For this review, take the finished solid that the model builds, in its own axes (mm). Face numbers are marked on the shaded views. A direction names the side the tool comes from. Coordinates: 2 decimals unless noted, no trailing zeros. Write each loop counter-clockwise with the first axis right and the second up, starting at its lowest first coordinate (ties: lowest second). Pieces come first, ordered by that corner, then holes.
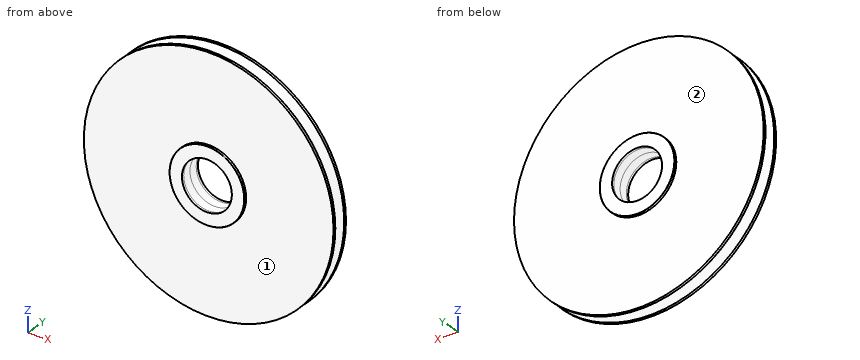
```python
from build123d import *
from build123d import SkipClean  # not in build123d's __all__

# Parameters (mm, degrees)
F0_R     = 50
F1_DEPTH = 3.5
F2_SIZE  = 2.5
F3_R     = 10.0003114876
F4_DEPTH = 3.5
F6_R     = 15
F6_R_2   = 10.0003114876
F7_DEPTH = 1
F8_R     = 15.0083101608
F8_R_2   = 10.0003114876
F9_DEPTH = 1
F10_R    = 0.1


with BuildPart() as f1:
    # F0 (on Front) → F1 (new body)
    with BuildSketch(Plane.XZ):
        Circle(F0_R)
    extrude(amount=F1_DEPTH)

    # F2
    f2_edges = [f1.edges().sort_by_distance(p)[0] for p in [
        (-50, -3.5, 0),
    ]]
    chamfer(f2_edges, length=F2_SIZE)

    # F3 (on face) → F4 (cut)
    with BuildSketch(Plane(origin=(0, 0, 0), x_dir=(-1, 0, 0), z_dir=(0, 1, 0))):
        Circle(F3_R)
    extrude(amount=-F4_DEPTH, mode=Mode.SUBTRACT)

    # F5: F1 across face


with BuildPart() as f1_1:
    add(f1.part, clean=False)
    add(f1.part.mirror(Plane.XZ.offset(3.5)), clean=False)

    # F6 (on face) → F7 (join)
    with BuildSketch(Plane.XZ.offset(7)):
        Circle(F6_R)
        Circle(F6_R_2, mode=Mode.SUBTRACT)
    with SkipClean():  # cleaning this boolean's faces spoils the solid; the shape is the same uncleaned
        extrude(amount=F7_DEPTH)

    # F8 (on face) → F9 (join)
    with BuildSketch(Plane(origin=(0, 0, 0), x_dir=(-1, 0, 0), z_dir=(0, 1, 0))):
        Circle(F8_R)
        Circle(F8_R_2, mode=Mode.SUBTRACT)
    extrude(amount=F9_DEPTH)

    # F10
    f10_edges = [f1_1.edges().sort_by_distance(p)[0] for p in [
        (-15, -8, 0),
        (15.00831, 1, 0),
    ]]
    fillet(f10_edges, radius=F10_R)


solid = f1_1.part
```
1) For L1, parallel to Z at x = 0, y = 0.55; L2, parallel to Y at x = 35.5, z = 24.5; L3, parallel to Z at x = 0, y = -6.2, list the stretches that pass through material, from the lowest coordinate up.
2) Clearance check with flat-ended pins moving along their axes: P1, Ø1, axis at x = 1.5, z = 21, coming from the +Y side; P2, Ø1, axis at x = 24.5, y = -2.5, coming from the +Z side; P3, Ø3, axis at x = 36.5, y = -2, coming from the -Z side. State where each tip first meets the part, or that it passes through.
3) Consider section A-A (z = 0). Give the boundary of the cut face in (x, y).
4) Tool access review of the marked faces 1 and 2: name each direction out of +Z, -Z, +X, -X, +Y, -Y from which nothing blocks a thin tool from reaching the whole face with its end or side.
5) Consider section B-B (x = 0). Give the boundary of the cut face in (y, z).
Results:
1. L1: z = -15.01 to -10, 10 to 15.01
1. L2: y = -7 to 0
1. L3: z = -50 to -10, 10 to 50
2. P1: stops at y = 0
2. P2: stops at z = 42.5
2. P3: stops at z = -35.33
3. outline: (-50, -7) - (-15, -7) - (-15, -7.9) arc R0.1 ccw to (-14.9, -8) - (-10, -8) - (-10, 1) - (-14.91, 1) arc R0.1 ccw to (-15.01, 0.9) - (-15.01, 0) - (-50, 0) - (-50, -1) - (-47.5, -3.5) - (-50, -6) - close; (10, -8) - (14.9, -8) arc R0.1 ccw to (15, -7.9) - (15, -7) - (50, -7) - (50, -6) - (47.5, -3.5) - (50, -1) - (50, 0) - (15.01, 0) - (15.01, 0.9) arc R0.1 ccw to (14.91, 1) - (10, 1) - close
4. face 1: -Y
4. face 2: +Y
5. outline: (-8, -14.9) arc R0.1 ccw to (-7.9, -15) - (-7, -15) - (-7, -50) - (-6, -50) - (-3.5, -47.5) - (-1, -50) - (0, -50) - (0, -15.01) - (0.9, -15.01) arc R0.1 ccw to (1, -14.91) - (1, -10) - (-8, -10) - close; (-8, 10) - (1, 10) - (1, 14.91) arc R0.1 ccw to (0.9, 15.01) - (0, 15.01) - (0, 50) - (-1, 50) - (-3.5, 47.5) - (-6, 50) - (-7, 50) - (-7, 15) - (-7.9, 15) arc R0.1 ccw to (-8, 14.9) - close
